Read the model definition and answer for the solid it produces. Units are mm, in the model's axes. A direction names the side the tool comes from. Give positions to 0.01 mm unless a question says otherwise; leave off trailing zeros. Write each loop counter-clockwise with the first axis right and the second up, starting at its lowest first coordinate (ties: lowest second). Pieces come first, ordered by that corner, then holes. Notation, with made-up numbers: (-31, 47) -> (4, 47) arc R20 cw to (4, 62) -> close; hole circle Ø11 at (87, 81.25). An arc over 180 degrees is marked (long way). Use a Markdown table: item, result.
from build123d import *

# Parameters (mm, degrees)
F0_R      = 7.874
F1_DEPTH  = 30.48
F3_D      = 3.5687
F2_R      = 2.3876
F4_DEPTH  = 3.81
F6_R      = 3.175
F7_DEPTH  = 12.7
F9_D      = 3.9878
F9_DEPTH  = 6.35
F9_TIP    = 1.1980559883
F10_SIZE2 = 0.508
F10_SIZE  = 0.508


with BuildPart() as f1:
    # F0 (on Front) → F1 (new body)
    with BuildSketch(Plane.XZ):
        with BuildLine():
            Line((-40.0582700968, 20.666185411), (-40.0582700968, 14.3161859534))
            Line((-40.0582700968, 14.3161859534), (4.3917299032, 14.3161859534))
            Line((4.3917299032, 14.3161859534), (4.3917299032, 20.666185411))
            Line((4.3917299032, 20.666185411), (1.7247299032, 20.666185411))
            ThreePointArc((1.7247299032, 20.666185411), (-2.7653981573, 22.5260573505), (-4.6252700968, 27.016185411))
            Line((-4.6252700968, 27.016185411), (-4.6252700968, 28.5401859534))
            ThreePointArc((-4.6252700968, 28.5401859534), (-7.4522754448, 35.3651806054), (-14.2772700968, 38.1921859534))
            Line((-14.2772700968, 38.1921859534), (-21.1352700968, 38.1921859534))
            ThreePointArc((-21.1352700968, 38.1921859534), (-27.9602647488, 35.3651806054), (-30.7872700968, 28.5401859534))
            Line((-30.7872700968, 28.5401859534), (-30.7872700968, 27.016185411))
            ThreePointArc((-30.7872700968, 27.016185411), (-32.6471420362, 22.5260573505), (-37.1372700968, 20.666185411))
            Line((-37.1372700968, 20.666185411), (-40.0582700968, 20.666185411))
        make_face()
        with Locations((-17.7062700968, 27.0161859534)):
            Circle(F0_R, mode=Mode.SUBTRACT)
    extrude(amount=F1_DEPTH)

    # F3 (through all)
    with Locations(Plane(origin=(0, 0, 14.3161859534), x_dir=(1, 0, 0), z_dir=(0, 0, -1))):
        with Locations((-33.7082700968, 24.13), (-33.7082700968, 6.35), (-1.9582700968, 24.13), (-1.9582700968, 6.35)):
            Hole(F3_D / 2)

    # F2 (on face) → F4 (cut)
    with BuildSketch(Plane(origin=(0, 0, 14.3161859534), x_dir=(1, 0, 0), z_dir=(0, 0, -1))):
        with Locations((-33.7082700968, 24.13)):
            Circle(F2_R)
        with Locations((-1.9582700968, 6.35)):
            Circle(F2_R)
        with Locations((-33.7082700968, 6.35)):
            Circle(F2_R)
        with Locations((-1.9582700968, 24.13)):
            Circle(F2_R)
    extrude(amount=-F4_DEPTH, mode=Mode.SUBTRACT)

    # F6 (on offset) → F7 (cut)
    with BuildSketch(Plane.XY.offset(33.366185411)):
        with Locations((-33.7082700968, -6.35)):
            Circle(F6_R)
        with Locations((-33.7082700968, -24.13)):
            Circle(F6_R)
        with Locations((-1.9582700968, -6.35)):
            Circle(F6_R)
        with Locations((-1.9582700968, -24.13)):
            Circle(F6_R)
    extrude(amount=-F7_DEPTH, mode=Mode.SUBTRACT)

    # F9
    with Locations(Plane.XY.offset(38.1921859534)):
        with Locations((-17.7062700968, -6.35), (-17.7062700968, -24.13)):
            Hole(F9_D / 2, depth=F9_DEPTH)
            with Locations((0, 0, -(F9_DEPTH + F9_TIP / 2))):  # 118° drill point
                Cone(0, F9_D / 2, F9_TIP, mode=Mode.SUBTRACT)

    # F10
    f10_edges = [f1.edges().sort_by_distance(p)[0] for p in [
        (-25.58027, 0, 27.016186),
    ]]
    chamfer(f10_edges, length=F10_SIZE, length2=F10_SIZE2)


solid = f1.part
Item 1: A tool of negligible diameter and unlimited length cuts with its end or side. For faces 1 (the face through (-4.625, -15, 28)), 2 (the face through (-15.714, -6.262, 36.384)), 3 (the face through (-2.48, -4.02, 16.19)), from which of +Z, -Z, +X, -X, +Y, -Y can it reach the whole face along a straight path? Write none if from no direction.
Return value:
| item | result |
|---|---|
| face 1 | +Z, +X, +Y, -Y |
| face 2 | +Z |
| face 3 | -Z |
Item 2: A cutting plane is placed at B-B (x = -1). Give the vertices of the cut face in (y, z), then the cut area to 3 significant figures.
Return value:
| item | result |
|---|---|
| outline | (-30.48, 14.32) -> (-26.32, 14.32) -> (-26.32, 18.13) -> (-25.64, 18.13) -> (-25.64, 20.67) -> (-27.16, 20.67) -> (-27.16, 21.28) -> (-30.48, 21.28) -> close; (-22.62, 18.13) -> (-21.94, 18.13) -> (-21.94, 14.32) -> (-8.54, 14.32) -> (-8.54, 18.13) -> (-7.86, 18.13) -> (-7.86, 20.67) -> (-9.38, 20.67) -> (-9.38, 21.28) -> (-21.1, 21.28) -> (-21.1, 20.67) -> (-22.62, 20.67) -> close; (-4.84, 18.13) -> (-4.16, 18.13) -> (-4.16, 14.32) -> (0, 14.32) -> (0, 21.28) -> (-3.32, 21.28) -> (-3.32, 20.67) -> (-4.84, 20.67) -> close |
| area | 156 mm^2 |
Item 3: A cutting plane is placed at A-A (y = -19.5). Give the vertices of the cut face in (x, z), then the cut area to 3 significant figures.
Return value:
| item | result |
|---|---|
| outline | (-40.06, 14.32) -> (4.39, 14.32) -> (4.39, 20.67) -> (1.72, 20.67) arc R6.35 cw to (-4.63, 27.02) -> (-4.63, 28.54) arc R9.65 ccw to (-14.28, 38.19) -> (-21.14, 38.19) arc R9.65 ccw to (-30.79, 28.54) -> (-30.79, 27.02) arc R6.35 cw to (-37.14, 20.67) -> (-40.06, 20.67) -> close; hole circle Ø15.75 at (-17.71, 27.02) |
| area | 523 mm^2 |
Item 4: Each of these flat-tipped pins is pushed along its axis until it touches: P1, Ø1.5, axis at y = -4.5, z = 32, coming from the -X side; P2, Ø12, axis at y = -6, z = 31.5, coming from the -X side; P3, Ø1.5, axis at x = -39, y = -9.5, coming from the +Z side. Where does it stop, or does it pass through?
Return value:
| item | result |
|---|---|
| P1 | x = -30.4 |
| P2 | x = -30.94 |
| P3 | z = 20.67 |
Item 5: For a pull along Y with two mould halves and no side action, classify faces 4 (the face through (-18, -30.48, 18)), 5 (the face through (-30.55, -23.81, 24.23)), 6 (the face through (-4.625, -2, 28)) as +Y half, -Y half, draft (parallel to the pull), parting line (faces both ways), or undercut.
Return value:
| item | result |
|---|---|
| face 4 | -Y half |
| face 5 | undercut |
| face 6 | draft |
Item 6: A cutting plane is placed at C-C (y = -24.13). Count the separate pieces of the cut face and the enclosed holes in it, then the cut area to 3 significant figures.
Return value:
| item | result |
|---|---|
| separate pieces | 3 |
| enclosed holes | 0 |
| area | 431 mm^2 |
Item 7: Straight lines are drawn through the part: line 1 along X through (y, z) = (-24.13, 18.75); line 2 along X through (y, z) = (-24.13, 15.8); line 3 along X through (y, z) = (-4.5, 27). For each, find the intervals that lie inside material, in ascending order. Write a range as [from, to].
Return value:
| item | result |
|---|---|
| line 1 | [-40.06, -35.49], [-31.92, -3.74], [-0.17, 4.39] |
| line 2 | [-40.06, -36.1], [-31.32, -4.35], [0.43, 4.39] |
| line 3 | [-30.79, -25.58], [-9.83, -4.63] |
